Input: dimensioned drawing with shaded views. Units: mm. Origin: part minimum x, y, z. A direction names the side the tool comes from. Give positions to 0.01 mm unless a question says otherwise; leave off trailing zeros. Write each loop counter-clockwise with the first axis right and the second up, starting at its lowest first coordinate (ties: lowest second). Pieces come first, ordered by that corner, then holes. Notation, with made-up numbers: M 26.5,55 L 49.5,55 A22 ccw 49.5,61 Z; hole C 64.25,86.5 d3. An arc over 180 degrees is marked long. Use CSV: the item, a comma, the result in double quotes. Start each with the question number.
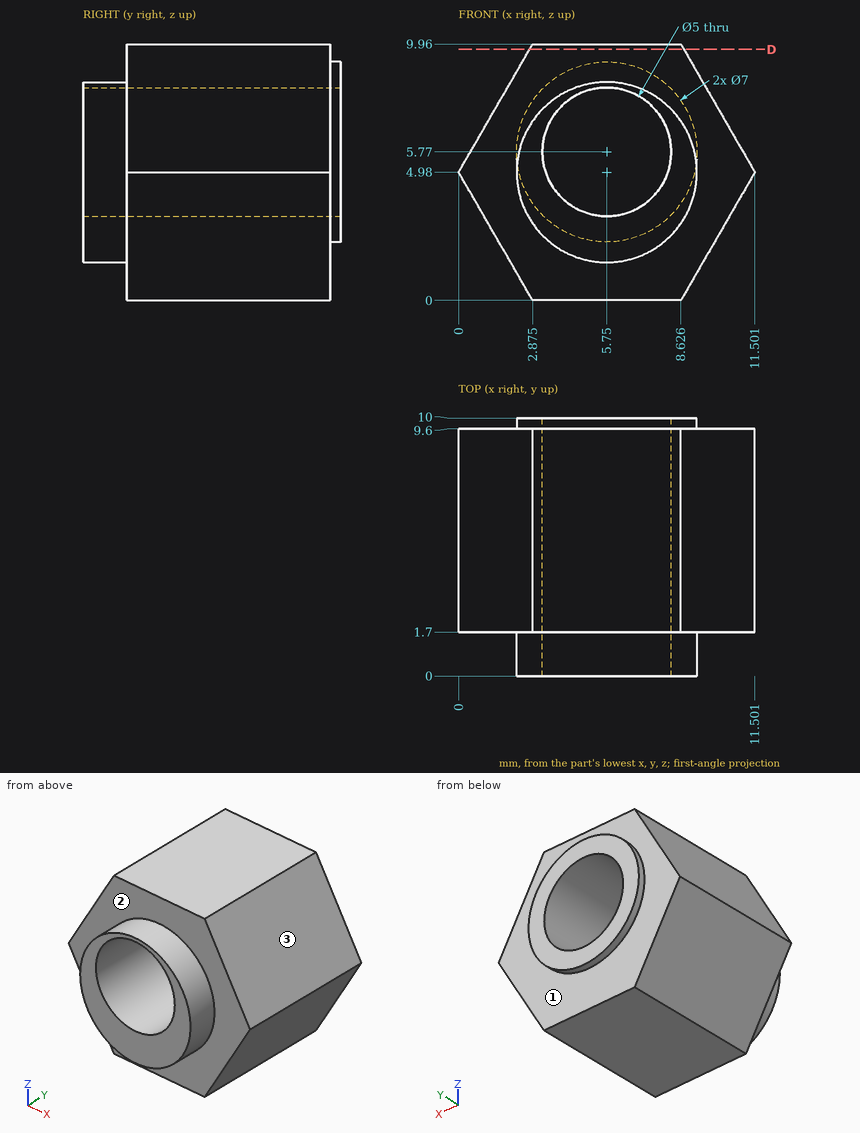
Item 1: Set-up query: the marked faces 1, 2 and 3. Return all of +Z, -Z, +X, -X, +Y, -Y with unobstructed straight access to the full face (end or side cutting, diameter ignored); none if empty.
Item 2: Section D-D (z = 9.75). Return the cut outline in (x, y).
Item 3: Contact query for flat-ended pins moving along their axis: pin 1 Ø1.5 at (y, z) = (4.5, 3) entering from -X; pin 2 Ø4.5 at (x, z) = (5.75, 5.77) entering from -Y; pin 3 Ø1.5 at (y, z) = (6.5, 9) entering from -X. Output: stop coordinate, or through.
Item 4: Material intervals for probe 1 along Y at (x, z) = (4, 1.25); probe 2 along X at (y, z) = (6.5, 4.5) (1 decimal); probe 3 along Z at (x, y) = (6, 5.5), sorted ascending.
Output values:
1,face 1,"+Y"
1,face 2,"-Y"
1,face 3,"+Z, +X, +Y, -Y"
2,outline,"M 2.75,1.7 L 8.75,1.7 L 8.75,9.6 L 2.75,9.6 Z"
3,pin 1,"stops at x = 0.71"
3,pin 2,"passes through"
3,pin 3,"stops at x = 1.89"
4,probe 1,"y = 1.7 to 9.6"
4,probe 2,"x = 0.3 to 3.6, 7.9 to 11.2"
4,probe 3,"z = 0 to 3.28, 8.26 to 9.96"
